The listing builds one solid part. Answer for the finished solid, in the listing's coordinates (mm). Face numbers are marked on the shaded views. A direction names the side the tool comes from. Round coordinates to 2 decimals unless told otherwise and drop trailing zeros. Write each loop counter-clockwise with the first axis right and the second up, starting at its lowest first coordinate (ties: lowest second). Pieces come first, ordered by that corner, then holes.
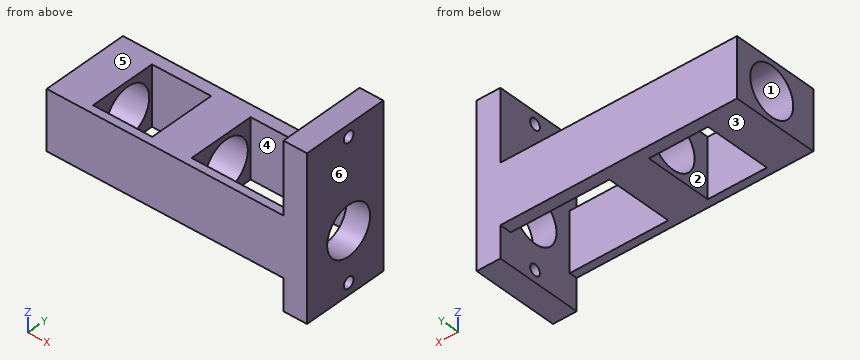
Autodesk Inventor part; units mm, degrees
ref_plane "YZ Plane" through (0, 0, 0) normal (1, 0, 0) x (0, 1, 0)
ref_plane "XZ Plane" through (0, 0, 0) normal (0, 1, 0) x (-1, 0, 0)
ref_plane "XY Plane" through (0, 0, 0) normal (0, 0, 1) x (1, 0, 0)
sketch "Sketch1" plane through (0, 0, 0) normal (1, 0, 0) x (0, 1, 0)
  line L0 (0, 0) -> (22, 0)
  line L1 (22, 0) -> (22, -41)
  line L2 (22, -41) -> (0, -41)
  line L3 (0, -41) -> (0, 0)
  line L4 (0, -22) -> (0, -32)
  line L5 (22, -33) -> (22, -23)
  circle A0 centre (12, -25.5) radius 6.2
  line L6 (22, -18) -> (0, -18)
  line L7 (0, -18) -> (0, -33)
  line L8 (0, -33) -> (22, -33)
  line L9 (22, -33) -> (22, -18)
  circle A1 centre (12, -3) radius 1.4
  circle A2 centre (12, -38) radius 1.4
  line L10 (19, -18) -> (2, -18)
  line L11 (2, -18) -> (2, -33)
  line L12 (2, -33) -> (19, -33)
  line L13 (19, -33) -> (19, -18)
  point P0 (0, -18)
  dimension "d10" = 41
  dimension "d11" = 22
  dimension "d12" = 15
  dimension "d15" = 10
  dimension "d17" = 8
  dimension "d18" = 2.8
  dimension "d19" = 2.8
  dimension "d20" = 12.4
  dimension "d22" = 10
  dimension "d23" = 10
  dimension "d24" = 35
  dimension "d25" = 3
  dimension "d26" = 7.5
  dimension "d27" = 17
  dimension "d28" = 3
extrude "Extrusion5" add sketch "Sketch1" along normal blind 6
extrude "Extrusion6" add sketch "Sketch1" against normal blind 50 contours L6 L11 L8 L3 | L1 L8 L13 L6
sketch "Sketch4" plane through (-50, 0, 0) normal (-1, 0, 0) x (0, 0, 1)
  line L0 (-41, 22) -> (-33, 22)
  line L1 (-33, 22) -> (-18, 22)
  line L2 (-18, 22) -> (-18, 0)
  line L3 (-18, 0) -> (-33, 0)
  line L4 (-33, 0) -> (-33, 22)
  circle A0 centre (-25.5, 12) radius 6.2
  circle A1 centre (-25.5, 12) radius 6.2
  point P0 (0, 0)
  dimension "d38" = 12.4
extrude "Extrusion7" add sketch "Sketch4" along normal blind 10
ref_plane "Work Plane1" through (-25, 0, 0) normal (1, 0, 0) x (0, 0, -1)
sketch "Sketch5" plane through (-25, 0, 0) normal (1, 0, 0) x (0, 0, -1)
  point P0 (0, 0)
sketch "Sketch6" plane through (-25, 0, 0) normal (1, 0, 0) x (0, 0, -1)
  circle A0 centre (25.5, 12) radius 6.2
  circle A1 centre (25.5, 12) radius 6.2
  line L0 (18, 2) -> (18, 19)
  line L1 (33, 0) -> (33, 2)
  line L2 (18, 19) -> (33, 19)
  line L3 (33, 19) -> (33, 2)
  line L4 (33, 2) -> (18, 2)
  line L5 (18, 2) -> (18, 19)
  point P0 (0, 0)
  point P1 (18, 2)
  dimension "d39" = 12.4
extrude "Extrusion8" add sketch "Sketch6" against normal blind 10
equation "\"d26\" = 0.5 * d12"
properties part number "_3DPrint"
1. Given pin 1 (10 mm diameter, centred on x = -11.5, y = 15.5, fed in from +Z); pin 2 (1.5 mm diameter, centred on y = 18, z = -6, fed in from -X), each flat-ended and moving along its own axis, determine where each tip first touches the part or whether it passes through.
Geometry says:
pin 1: stops at z = -18
pin 2: stops at x = 0
2. For a pull along X with two mould halves and no side action, classify the marked faces 4, 5 and 6 as released by +X, released by -X, zero draft, split by the parting line, or undercut.
Geometry says:
face 4: undercut
face 5: zero draft
face 6: released by +X
3. Section A-A on z = -38 is taken. Determine the outline of the cut face in (x, y).
Geometry says:
outline: (0, 0) - (6, 0) - (6, 10.6) - (0, 10.6) - close; (0, 13.4) - (6, 13.4) - (6, 22) - (0, 22) - close
4. Section B-B on x = -42.5 is taken. Determine the outline of the cut face in (y, z).
Geometry says:
outline: (0, -33) - (2, -33) - (2, -18) - (0, -18) - close; (19, -33) - (22, -33) - (22, -18) - (19, -18) - close
5. Section C-C on y = 12 is taken. Give the number of separate pieces and of enclosed holes in the cut face, plus the area to 3 significant figures.
Geometry says:
separate pieces: 8
enclosed holes: 0
area: 190 mm2
6. A tool of negligible diameter and unlimited length cuts with its end or side. For the marked faces 1, 2 and 3, from which of +Z, -Z, +X, -X, +Y, -Y can it reach the whole face along a straight path? Write none if from no direction.
Geometry says:
face 1: +X, -X
face 2: +Z, -Z
face 3: -Z, -X, +Y, -Y
7. Straight lines are drawn through the part: line 1 along X through (y, z) = (5.5, -21); line 2 along Z through (x, y) = (2.35, 12); line 3 along Y through (x, z) = (-29, -25.5). For each, find the intervals that lie inside material, in ascending order.
Geometry says:
line 1: x = -60 to -50, -35 to -25, 0 to 6
line 2: z = -41 to -39.4, -36.6 to -31.7, -19.3 to -4.4, -1.6 to 0
line 3: y = 0 to 5.8, 18.2 to 22
8. Section D-D on y = 3.5 is taken. Determine the outline of the cut face in (x, z), plus the area to 3 significant figures.
Geometry says:
outline: (-60, -33) - (-50, -33) - (-50, -18) - (-60, -18) - close; (-35, -33) - (-25, -33) - (-25, -18) - (-35, -18) - close; (0, -41) - (6, -41) - (6, 0) - (0, 0) - close
area: 546 mm2
